CAD build for the part. Positions are in the model's coordinates, mm. A direction names the side the tool comes from. Coordinates: 2 decimals unless noted, no trailing zeros. Order: outer loops, then holes, each group sorted by start corner. A loop starts at its lowest first (then second) coordinate and runs counter-clockwise, first axis right, second up. Notation, with made-up numbers: M 38.25,73.5 L 90.25,73.5 A13 ccw 90.25,81.5 Z; hole C 78.5,37 d11. An arc over 180 degrees is marked long. Write item = value, one per line.
from build123d import *

# Parameters (mm, degrees)
SKETCH1_W            = 136
SKETCH1_H            = 95
BOSS_EXTRUDE1_DEPTH  = 15
SKETCH2_W            = 128
SKETCH2_H            = 86
CUT_EXTRUDE1_DEPTH   = 7
SNAP_START           = 64
SNAP_HOOK2_DEPTH     = 2
SNAP_HOOK2_2_DEPTH   = 2
FILLET1_R            = 1
FILLET2_R            = 0.5
FILLET2_OF_MIRROR1_R = 0.5
SNAP_START_2         = 43.25
SNAP_HOOK3_DEPTH     = 2
FILLET3_R            = 0.5
FILLET3_OF_MIRROR2_R = 0.5


with BuildPart() as part:
    # Sketch1 → Boss-Extrude1 (new body)
    with BuildSketch(Plane(origin=(0, 0, 0), x_dir=(1, 0, 0), z_dir=(0, 1, 0))):
        Rectangle(SKETCH1_W, SKETCH1_H)
    extrude(amount=BOSS_EXTRUDE1_DEPTH)

    # Sketch2 → Cut-Extrude1 (cut)
    with BuildSketch(Plane(origin=(0, 15, 0), x_dir=(1, 0, 0), z_dir=(0, 1, 0))):
        Rectangle(SKETCH2_W, SKETCH2_H)
    extrude(amount=-CUT_EXTRUDE1_DEPTH, mode=Mode.SUBTRACT)



with BuildPart() as body_2:
    # Snap Hook2: read off the stored shape, not the designer's step
    # Snap Hook2 outline → Snap Hook2 (new body)
    with BuildSketch(Plane.YZ.offset(SNAP_START)):
        Polygon((21, -2), (21, 2), (18, 2.157223338), (18, -2.157223338), align=None)
    snap_hook2 = extrude(amount=SNAP_HOOK2_DEPTH)


with BuildPart() as part_1:
    add(part.part)

    add(body_2.part)  # Snap Hook2 2 merges body 2
    # Snap Hook2 2 outline → Snap Hook2 2 (add)
    with BuildSketch(Plane.YZ.offset(SNAP_START)):
        Polygon((18, -2.157223338), (18, 2.157223338), (15, 2.314446676), (15, -2.314446676), align=None)
    snap_hook2_2 = extrude(amount=SNAP_HOOK2_2_DEPTH)

    # Snap Hook2 3: loft between two sections, ruled curve by curve
    snap_hook2_3_from = [
        Edge.make_line((66, 21, -2), (66, 21, 2)),
        Edge.make_line((66, 18, 2.157223338), (66, 18, -2.157223338)),
        Edge.make_line((66, 18, 2.157223338), (66, 21, 2)),
        Edge.make_line((66, 18, -2.157223338), (66, 21, -2)),
    ]
    snap_hook2_3_to = [
        Edge.make_line((68, 19, -2.104815559), (68, 19, 2.104815559)),
        Edge.make_line((68, 18, 2.157223338), (68, 18, -2.157223338)),
        Edge.make_line((68, 18, 2.157223338), (68, 19, 2.104815559)),
        Edge.make_line((68, 18, -2.157223338), (68, 19, -2.104815559)),
    ]
    snap_hook2_3 = Solid(Shell([*[Face.make_surface_from_curves(snap_hook2_3_from[k], snap_hook2_3_to[k]) for k in range(4)], Face(Wire(snap_hook2_3_from)), Face(Wire(snap_hook2_3_to))]))
    add(snap_hook2_3)

    # Fillet1
    fillet1_edges = [part_1.edges().sort_by_distance(p)[0] for p in [
        (-64, 11.5, 43),
        (-64, 11.5, -43),
        (64, 11.5, -43),
        (64, 11.5, 43),
        (68, 7.5, 47.5),
        (68, 7.5, -47.5),
        (-68, 7.5, -47.5),
        (-68, 7.5, 47.5),
    ]]
    fillet(fillet1_edges, radius=FILLET1_R)

    # Fillet2
    fillet2_edges = [part_1.edges().sort_by_distance(p)[0] for p in [
        (66, 15, 0),
    ]]
    fillet(fillet2_edges, radius=FILLET2_R)

    # Mirror1: Snap Hook2, Snap Hook2 2, Snap Hook2 3 across plane
    add(snap_hook2.mirror(Plane(origin=(0, 0, 0), x_dir=(0, 0, 1), z_dir=(1, 0, 0))))
    add(snap_hook2_2.mirror(Plane(origin=(0, 0, 0), x_dir=(0, 0, 1), z_dir=(1, 0, 0))))
    add(snap_hook2_3.mirror(Plane(origin=(0, 0, 0), x_dir=(0, 0, 1), z_dir=(1, 0, 0))))

    # Fillet2 of Mirror1
    fillet2_of_mirror1_edges = [part_1.edges().sort_by_distance(p)[0] for p in [
        (-66, 15, 0),
    ]]
    fillet(fillet2_of_mirror1_edges, radius=FILLET2_OF_MIRROR1_R)

    # Snap Hook3: read off the stored shape, not the designer's step
    # Snap Hook3 outline → Snap Hook3 (add)
    with BuildSketch(Plane.XY.offset(SNAP_START_2)):
        Polygon((2, 21), (-2, 21), (-2.314446676, 15), (2.314446676, 15), align=None)
    snap_hook3 = extrude(amount=SNAP_HOOK3_DEPTH)

    # Snap Hook3 2: loft between two sections, ruled curve by curve
    snap_hook3_2_from = [
        Edge.make_line((-2.157223338, 18, 45.25), (2.157223338, 18, 45.25)),
        Edge.make_line((2, 21, 45.25), (-2, 21, 45.25)),
        Edge.make_line((2, 21, 45.25), (2.157223338, 18, 45.25)),
        Edge.make_line((-2, 21, 45.25), (-2.157223338, 18, 45.25)),
    ]
    snap_hook3_2_to = [
        Edge.make_line((-2.157223338, 18, 47.25), (2.157223338, 18, 47.25)),
        Edge.make_line((2.104815559, 19, 47.25), (-2.104815559, 19, 47.25)),
        Edge.make_line((2.104815559, 19, 47.25), (2.157223338, 18, 47.25)),
        Edge.make_line((-2.104815559, 19, 47.25), (-2.157223338, 18, 47.25)),
    ]
    snap_hook3_2 = Solid(Shell([*[Face.make_surface_from_curves(snap_hook3_2_from[k], snap_hook3_2_to[k]) for k in range(4)], Face(Wire(snap_hook3_2_from)), Face(Wire(snap_hook3_2_to))]))
    add(snap_hook3_2)

    # Fillet3
    # the kernel refuses this fillet: 0.5 mm, written as the material it adds along each edge
    with BuildSketch(Plane(origin=(-3.564446676, 15, 45.25), x_dir=(0, 0, 1), z_dir=(1, 0, 0))) as fillet3_piece_1_section:
        with BuildLine():
            CenterArc((FILLET3_R, -FILLET3_R), FILLET3_R, 90, 90)
            Line((0, -FILLET3_R), (-FILLET3_R * 0.02, -FILLET3_R))
            Line((-FILLET3_R * 0.02, -FILLET3_R), (-FILLET3_R * 0.02, FILLET3_R * 0.02))
            Line((-FILLET3_R * 0.02, FILLET3_R * 0.02), (FILLET3_R, FILLET3_R * 0.02))
            Line((FILLET3_R, FILLET3_R * 0.02), (FILLET3_R, 0))
        make_face()
    fillet3_piece_1 = extrude(amount=7.128893352, mode=Mode.PRIVATE)
    fillet3_piece_1 = split(fillet3_piece_1, bisect_by=Plane(origin=(2.29834408, 15.307255844, 45.25), z_dir=(-0.998629534751949, -0.05233595629302951, 0)), keep=Keep.TOP, mode=Mode.PRIVATE)
    fillet3_piece_1 = split(fillet3_piece_1, bisect_by=Plane(origin=(-2.317870491, 14.93466971, 45.25), z_dir=(0.998629534751949, -0.05233595629302951, 0)), keep=Keep.TOP, mode=Mode.PRIVATE)
    add(fillet3_piece_1)
    with BuildSketch(Plane(origin=(-3.396978431, 15, 43.25), x_dir=(0, 0, -1), z_dir=(1, 0, 0))) as fillet3_piece_2_section:
        with BuildLine():
            CenterArc((0.5, 0.433012702), FILLET3_R, 180, 60)
            Line((0, 0.433012702), (-0.01, 0.433012702))
            Line((-0.01, 0.433012702), (-0.01, 0))
            Line((-0.01, 0), (0, -0.01))
            ThreePointArc((0, -0.01), (0.125, -0.01), (0.245, -0.008660254))
            Line((0.245, -0.008660254), (0.25, 0))
        make_face()
    fillet3_piece_2 = extrude(amount=6.793956861, mode=Mode.PRIVATE)
    fillet3_piece_2 = split(fillet3_piece_2, bisect_by=Plane(origin=(2.298802784, 15.298503245, 43.25), z_dir=(-0.998629534751949, -0.05233595629302951, 0)), keep=Keep.TOP, mode=Mode.PRIVATE)
    fillet3_piece_2 = split(fillet3_piece_2, bisect_by=Plane(origin=(-2.317411787, 14.94342231, 43.25), z_dir=(0.998629534751949, -0.05233595629302951, 0)), keep=Keep.TOP, mode=Mode.PRIVATE)
    add(fillet3_piece_2)

    # Mirror2: Snap Hook3, Snap Hook3 2 across plane
    add(snap_hook3.mirror(Plane.XY))
    add(snap_hook3_2.mirror(Plane.XY))

    # Fillet3 of Mirror2
    # the kernel refuses this fillet: 0.5 mm, written as the material it adds along each edge
    with BuildSketch(Plane(origin=(-3.564446676, 15, -45.25), x_dir=(0, 0, -1), z_dir=(1, 0, 0))) as fillet3_of_mirror2_piece_1_section:
        with BuildLine():
            CenterArc((FILLET3_OF_MIRROR2_R, FILLET3_OF_MIRROR2_R), FILLET3_OF_MIRROR2_R, 180, 90)
            Line((0, FILLET3_OF_MIRROR2_R), (-FILLET3_OF_MIRROR2_R * 0.02, FILLET3_OF_MIRROR2_R))
            Line((-FILLET3_OF_MIRROR2_R * 0.02, FILLET3_OF_MIRROR2_R), (-FILLET3_OF_MIRROR2_R * 0.02, -FILLET3_OF_MIRROR2_R * 0.02))
            Line((-FILLET3_OF_MIRROR2_R * 0.02, -FILLET3_OF_MIRROR2_R * 0.02), (FILLET3_OF_MIRROR2_R, -FILLET3_OF_MIRROR2_R * 0.02))
            Line((FILLET3_OF_MIRROR2_R, -FILLET3_OF_MIRROR2_R * 0.02), (FILLET3_OF_MIRROR2_R, 0))
        make_face()
    fillet3_of_mirror2_piece_1 = extrude(amount=7.128893352, mode=Mode.PRIVATE)
    fillet3_of_mirror2_piece_1 = split(fillet3_of_mirror2_piece_1, bisect_by=Plane(origin=(-2.317870491, 14.93466971, -45.25), z_dir=(0.998629534751949, -0.05233595629302951, 0)), keep=Keep.TOP, mode=Mode.PRIVATE)
    fillet3_of_mirror2_piece_1 = split(fillet3_of_mirror2_piece_1, bisect_by=Plane(origin=(2.29834408, 15.307255844, -45.25), z_dir=(-0.998629534751949, -0.05233595629302951, 0)), keep=Keep.TOP, mode=Mode.PRIVATE)
    add(fillet3_of_mirror2_piece_1)
    with BuildSketch(Plane(origin=(-3.396978431, 15, -43.25), x_dir=(0, 0, 1), z_dir=(1, 0, 0))) as fillet3_of_mirror2_piece_2_section:
        with BuildLine():
            CenterArc((0.5, -0.433012702), FILLET3_OF_MIRROR2_R, 120, 60)
            Line((0, -0.433012702), (-0.01, -0.433012702))
            Line((-0.01, -0.433012702), (-0.01, 0))
            Line((-0.01, 0), (0, 0.01))
            ThreePointArc((0, 0.01), (0.125, 0.01), (0.245, 0.008660254))
            Line((0.245, 0.008660254), (0.25, 0))
        make_face()
    fillet3_of_mirror2_piece_2 = extrude(amount=6.793956861, mode=Mode.PRIVATE)
    fillet3_of_mirror2_piece_2 = split(fillet3_of_mirror2_piece_2, bisect_by=Plane(origin=(-2.317411787, 14.94342231, -43.25), z_dir=(0.998629534751949, -0.05233595629302951, 0)), keep=Keep.TOP, mode=Mode.PRIVATE)
    fillet3_of_mirror2_piece_2 = split(fillet3_of_mirror2_piece_2, bisect_by=Plane(origin=(2.298802784, 15.298503245, -43.25), z_dir=(-0.998629534751949, -0.05233595629302951, 0)), keep=Keep.TOP, mode=Mode.PRIVATE)
    add(fillet3_of_mirror2_piece_2)


solid = part_1.part
(1) Pin check, flat tips, straight feed: pin 1 Ø1.3 at (x, y) = (-1, 17) entering from -Z; pin 2 Ø1.5 at (x, z) = (-16.5, 21) entering from +Y; pin 3 Ø1.2 at (y, z) = (16.5, 1) entering from +X. Stop position of each tip, or through.
Evaluation:
pin_1 = -45.25
pin_2 = 8
pin_3 = 66
(2) Tool access for faces 4 (the face through (64, 12, 1)), 5 (the face through (0, 18, 43.25)), 6 (the face through (-68, 7, 1)): list every direction of +Z, -Z, +X, -X, +Y, -Y with a clear straight run to the whole face (end or side of a thin tool).
Evaluation:
face_4 = +Y
face_5 = +X, -X, +Y
face_6 = +Z, -Z, -X, +Y, -Y
(3) Slice it at C-C, the plane z = -19.5. Write the cut outline in (x, y).
Evaluation:
outline = M -68,0 L 68,0 L 68,15 L 64,15 L 64,8 L -64,8 L -64,15 L -68,15 Z
(4) Slice it at A-A, the plane y = 11.5. Write the cut outline in (x, z).
Evaluation:
outline = M -68,-46.5 A1 ccw -67,-47.5 L 67,-47.5 A1 ccw 68,-46.5 L 68,46.5 A1 ccw 67,47.5 L -67,47.5 A1 ccw -68,46.5 Z; hole M -64,-42 A1 ccw -63,-43 L 63,-43 A1 ccw 64,-42 L 64,42 A1 ccw 63,43 L -63,43 A1 ccw -64,42 Z
(5) Wall check: line 1 (X direction, y = 8.5, z = 4); line 2 (Z direction, x = 14, y = 9); line 3 (Z direction, x = 1.5, y = 18.5). Give the ranges that are in metal, low to high. Write a range as from..to.
Evaluation:
line_1 = -68..-64, 64..68
line_2 = -47.5..-43, 43..47.5
line_3 = -47.25..-43.25, 43.25..47.25
(6) Pull direction Z, two halves, no side cores. Call faces 1 (the face through (-1, 7, 47.5)), 2 (the face through (-1, 7, -47.5)), 3 (the face through (0, 18, -43.25)): +Z half, -Z half, draft (parallel to the pull), parting line (faces both ways), or undercut.
Evaluation:
face_1 = +Z half
face_2 = -Z half
face_3 = undercut
(7) Slice it at B-B, the plane x = -46. Write the cut outline in (y, z), then the cut area to 3 significant figures.
Evaluation:
outline = M 0,-47.5 L 15,-47.5 L 15,-43 L 8,-43 L 8,43 L 15,43 L 15,47.5 L 0,47.5 Z
area = 823 mm²
